Part model, mm, in its own coordinate system. Face numbers are marked on the shaded views. Give positions to 0.01 mm unless a question says otherwise; leave off trailing zeros. Order: outer loops, then holes, each group sorted by start corner. A loop starts at its lowest first (then second) coordinate and runs counter-clockwise, first axis right, second up. Notation, with made-up numbers: M -25,-1 L 14,-1 A25 cw 14,28 Z; hole C 79,13 d1. An arc over 180 degrees is marked long. Return JSON: item names as keys, results as strings.
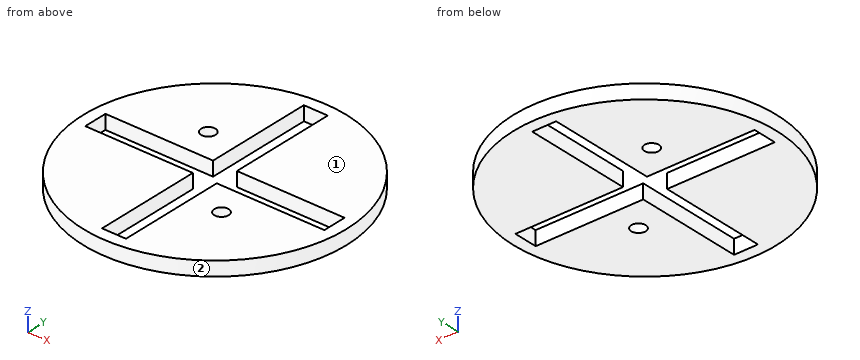
Autodesk Inventor part; units mm, degrees
ref_plane "YZ Plane" through (0, 0, 0) normal (1, 0, 0) x (0, 1, 0)
ref_plane "XZ Plane" through (0, 0, 0) normal (0, 1, 0) x (-1, 0, 0)
ref_plane "XY Plane" through (0, 0, 0) normal (0, 0, 1) x (1, 0, 0)
sketch "Sketch1" plane through (0, 0, 0) normal (0, 0, 1) x (1, 0, 0)
  circle A0 centre (0, 0) radius 27.5
  dimension "d0" = 55
extrude "Extrusion1" add sketch "Sketch1" along normal blind 3
sketch "Sketch2" plane through (0, 0, 0) normal (0, 0, -1) x (-1, 0, 0)
  circle A0 centre (0, 0) radius 27.5
  line L0 (-2.5, -25) -> (-2.5, 25)
  line L1 (-2.5, 25) -> (2.5, 25)
  line L2 (2.5, 25) -> (2.5, -25)
  line L3 (2.5, -25) -> (-2.5, -25)
  line L4 (-2.5, -25) -> (2.5, 25) construction
  line L5 (-2.5, 25) -> (2.5, -25) construction
  line L6 (-25, -2.5) -> (25, -2.5)
  line L7 (25, -2.5) -> (25, 2.5)
  line L8 (25, 2.5) -> (-25, 2.5)
  line L9 (-25, 2.5) -> (-25, -2.5)
  line L10 (-25, -2.5) -> (25, 2.5) construction
  line L11 (25, -2.5) -> (-25, 2.5) construction
  dimension "d3" = 50
  dimension "d4" = 5
  dimension "d5" = 50
  dimension "d6" = 5
extrude "Extrusion2" cut sketch "Sketch2" against normal up to next contours L0 L6 L2 L3 | L6 L9 L8 L0 | L0 L8 L2 L6 | L0 L1 L2 L8 | L2 L8 L7 L6
sketch "Sketch3" plane through (0, 0, 0) normal (0, 0, -1) x (-1, 0, 0)
  circle A0 centre (8.8388, 8.8388) radius 1.5
  circle A1 centre (-8.8388, -8.8388) radius 1.5
extrude "Extrusion3" cut sketch "Sketch3" against normal up to next
properties part number "TransparentTop"
Q1. Probe line 1 along X through (y, z) = (21, 2.6); line 2 along X through (y, z) = (4, 2.35); line 3 along Y through (x, z) = (-4.5, 2). List the from-to ranges inside material, lowest first.
Established:
{"line 1": "x = -17.76 to -2.5, 2.5 to 17.76", "line 2": "x = -27.21 to -2.5, 2.5 to 27.21", "line 3": "y = -27.13 to -2.5, 2.5 to 27.13"}
Q2. Pin check, flat tips, straight feed: pin 1 (0.9 mm diameter, centred on x = -1, z = 1.5, fed in from -Y); pin 2 (0.9 mm diameter, centred on x = 1, z = 1, fed in from +Y); pin 3 (0.9 mm diameter, centred on x = -9, z = 1, fed in from -Y); pin 4 (2.5 mm diameter, centred on x = -8.84, y = 8.84, fed in from +Z). Stop position of each tip, or through.
Established:
{"pin 1": "stops at y = -27.49", "pin 2": "stops at y = 27.49", "pin 3": "stops at y = -26.14", "pin 4": "passes through"}
Q3. Two-plate mould, pull along X, no slides. Class the marked faces 1 and 2: +X half, -X half, draft (parallel to the pull), parting line (faces both ways), or undercut.
Established:
{"face 1": "draft", "face 2": "parting line"}
Q4. Band-saw the part on A-A (y = 0). Give the cut face in (x, z).
Established:
{"outline": "M -27.5,0 L -25,0 L -25,3 L -27.5,3 Z; M 25,0 L 27.5,0 L 27.5,3 L 25,3 Z"}
Q5. Band-saw the part on C-C (z = 1.65). Give the cut face in (x, y), then the cut area to 3 significant figures.
Established:
{"outline": "C 0,0 d55; hole M -25,-2.5 L -2.5,-2.5 L -2.5,-25 L 2.5,-25 L 2.5,-2.5 L 25,-2.5 L 25,2.5 L 2.5,2.5 L 2.5,25 L -2.5,25 L -2.5,2.5 L -25,2.5 Z; hole C -8.84,8.84 d3; hole C 8.84,-8.84 d3", "area": "1,890 mm²"}
